Check sheet for the modelled part. Datum: model origin and axes. Units: mm. Face numbers are marked on the shaded views. A direction names the side the tool comes from. Round coordinates to 2 decimals unless told otherwise and drop trailing zeros. Write each loop counter-clockwise with the first axis right and the second up, starting at its lowest first coordinate (ties: lowest second). Pieces come first, ordered by that corner, then holes. Notation, with made-up numbers: (-31.5, -13.75) - (-15.5, -13.75) arc R13 cw to (-15.5, 6.25) - close; hole circle Ø2 at (-33, 21.5). An arc over 180 degrees is marked (long way). Use one line per item in the form item = value. Start each with the question number.
1) Section check D-D (y = 9.5). Record the boundary of the cut face in (x, z), then the cut area to 3 significant figures.
2) Scan lines: probe 1 along X at (y, z) = (21, 2.5); probe 2 along Y at (x, z) = (32, 6); probe 3 along X at (y, z) = (23.5, 4.75). Record each from-to range of solid material in increasing order.
3) Draft check along Y on the marked faces 1, 2 and 3. Enter one of: +Y half, -Y half, draft (parallel to the pull), parting line (faces both ways), or undercut.
4) Section check A-A (y = 3). Record the boundary of the cut face in (x, z).
5) Section check C-C (x = 28). Record the boundary of the cut face in (y, z), then the cut area to 3 significant figures.
6) Set-up check for the marked faces 4, 5, 6 and 7: record each of +Z, -Z, +X, -X, +Y, -Y from which the full face is reachable in a straight line by a thin tool's end or side.
7) Gauge pin test, flat ends, axial feed: P1, Ø1.5, axis at y = 33, z = 3, coming from the -X side; P2, Ø2.5, axis at y = 31.49, z = 5, coming from the +X side; P3, Ø2, axis at x = 26, z = 8, coming from the +Y side. Record the tip position at first contact, or that the pin passes through.
8) Section check B-B (x = 24). Record the boundary of the cut face in (y, z).
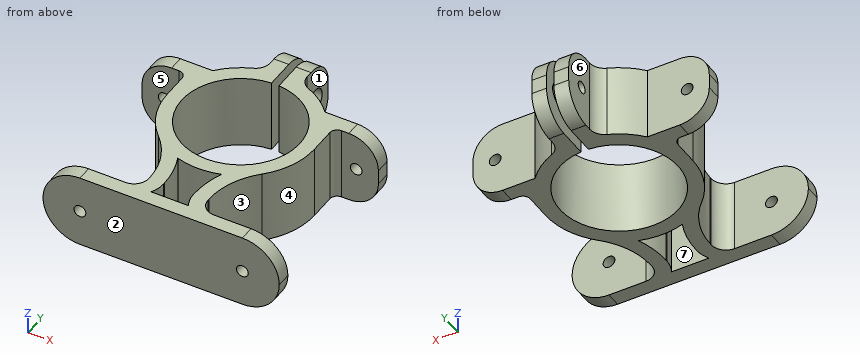
from build123d import *

# Parameters (mm, degrees)
BOSS_EXTRUDE1_DEPTH = 10
SKETCH3_R           = 0.8
CUT_EXTRUDE1_DEPTH  = 2
SKETCH4_R           = 0.8
CUT_EXTRUDE2_DEPTH  = 2
SKETCH5_R           = 0.8
CUT_EXTRUDE3_DEPTH  = 2
SKETCH6_R           = 0.8
CUT_EXTRUDE4_DEPTH  = 3
SKETCH7_R           = 1.6
CUT_EXTRUDE5_DEPTH  = 3
CUT_EXTRUDE6_DEPTH  = 10


with BuildPart() as part:
    # Sketch1 → Boss-Extrude1 (new body)
    with BuildSketch(Plane.XY):
        with BuildLine():
            Line((16.803004448, 0), (48.803096805, 0))
            Line((48.803096805, 0), (48.803096805, 2))
            Line((48.803096805, 2), (38.803096805, 2))
            ThreePointArc((38.803096805, 2), (37.388883243, 2.585786438), (36.803096805, 4))
            Line((36.803096805, 4), (36.803096805, 4.217123744))
            ThreePointArc((36.803096805, 4.217123744), (37.58355047, 8.090102619), (39.803089878, 11.358545383))
            ThreePointArc((39.803089878, 11.358545383), (42.022639537, 14.62700324), (42.803096805, 18.5))
            Line((42.803096805, 18.5), (42.803096805, 22))
            ThreePointArc((42.803096805, 22), (43.095990024, 22.707106781), (43.803096805, 23))
            Line((43.803096805, 23), (48.803096805, 23))
            Line((48.803096805, 23), (48.803096805, 25))
            Line((48.803096805, 25), (44.105786895, 25))
            Line((44.105786895, 25), (40.40245347, 25))
            ThreePointArc((40.40245347, 25), (38.644426823, 26.616603213), (36.553207437, 27.770234489))
            ThreePointArc((36.553207437, 27.770234489), (35.644914528, 28.506251313), (35.303235335, 29.624272825))
            Line((35.303235335, 29.624272825), (35.303235335, 34.487492178))
            Line((35.303235335, 34.487492178), (33.303050626, 34.487492178))
            Line((33.303050626, 34.487492178), (33.303050626, 26.484348185))
            ThreePointArc((33.303050626, 26.484348185), (32.803050626, 10.500011503), (32.303050626, 26.484348185))
            Line((32.303050626, 26.484348185), (32.303050626, 34.487492178))
            Line((32.303050626, 34.487492178), (30.303050626, 34.487492178))
            Line((30.303050626, 34.487492178), (30.303050626, 29.624347545))
            ThreePointArc((30.303050626, 29.624347545), (29.961362151, 28.506312265), (29.05304774, 27.770296755))
            ThreePointArc((29.05304774, 27.770296755), (26.961741815, 26.616651708), (25.203647783, 25))
            Line((25.203647783, 25), (21.500314358, 25))
            Line((21.500314358, 25), (16.803004448, 25))
            Line((16.803004448, 25), (16.803004448, 23))
            Line((16.803004448, 23), (21.803004448, 23))
            ThreePointArc((21.803004448, 23), (22.510111229, 22.707106781), (22.803004448, 22))
            Line((22.803004448, 22), (22.803004448, 18.5))
            ThreePointArc((22.803004448, 18.5), (23.583461716, 14.62700324), (25.803011375, 11.358545383))
            ThreePointArc((25.803011375, 11.358545383), (28.022550783, 8.090102619), (28.803004448, 4.217123744))
            Line((28.803004448, 4.217123744), (28.803004448, 4))
            ThreePointArc((28.803004448, 4), (28.21721801, 2.585786438), (26.803004448, 2))
            Line((26.803004448, 2), (16.803004448, 2))
            Line((16.803004448, 2), (16.803004448, 0))
        make_face()
        with BuildLine():
            Line((34.803096805, 4), (34.803096805, 4.217123744))
            ThreePointArc((34.803096805, 4.217123744), (35.049071096, 6.634328662), (35.776910074, 8.952438536))
            ThreePointArc((35.776910074, 8.952438536), (32.803050626, 8.500011503), (29.829191179, 8.952438536))
            ThreePointArc((29.829191179, 8.952438536), (30.557030157, 6.634328662), (30.803004448, 4.217123744))
            Line((30.803004448, 4.217123744), (30.803004448, 4))
            ThreePointArc((30.803004448, 4), (30.666707753, 2.96472382), (30.267106063, 2))
            Line((30.267106063, 2), (35.33899519, 2))
            ThreePointArc((35.33899519, 2), (34.9393935, 2.96472382), (34.803096805, 4))
        make_face(mode=Mode.SUBTRACT)
    extrude(amount=BOSS_EXTRUDE1_DEPTH)

    # Sketch3 → Cut-Extrude1 (cut)
    with BuildSketch(Plane(origin=(0, 2, 0), x_dir=(1, 0, 0), z_dir=(0, 1, 0))):
        with BuildLine():
            ThreePointArc((48.803096805, -5), (47.338630711, -8.535533906), (43.803096805, -10))
            Line((43.803096805, -10), (48.803096805, -10))
            Line((48.803096805, -10), (48.803096805, -5))
        make_face()
        with BuildLine():
            ThreePointArc((43.803096805, 0), (47.338630711, -1.464466094), (48.803096805, -5))
            Line((48.803096805, -5), (48.803096805, 0))
            Line((48.803096805, 0), (43.803096805, 0))
        make_face()
        with Locations(Location((43.803096805, -5, 0), (0, 0, 180))):
            Circle(SKETCH3_R)
    extrude(amount=-CUT_EXTRUDE1_DEPTH, mode=Mode.SUBTRACT)

    # Sketch4 → Cut-Extrude2 (cut)
    with BuildSketch(Plane(origin=(0, 2, 0), x_dir=(1, 0, 0), z_dir=(0, 1, 0))):
        with BuildLine():
            Line((16.803004448, -10), (21.803004448, -10))
            ThreePointArc((21.803004448, -10), (18.267470542, -8.535533906), (16.803004448, -5))
            Line((16.803004448, -5), (16.803004448, -10))
        make_face()
        with BuildLine():
            Line((16.803004448, 0), (16.803004448, -5))
            ThreePointArc((16.803004448, -5), (18.267470542, -1.464466094), (21.803004448, 0))
            Line((21.803004448, 0), (16.803004448, 0))
        make_face()
        with Locations(Location((21.803004448, -5, 0), (0, 0, 270))):
            Circle(SKETCH4_R)
    extrude(amount=-CUT_EXTRUDE2_DEPTH, mode=Mode.SUBTRACT)

    # Sketch5 → Cut-Extrude3 (cut)
    with BuildSketch(Plane(origin=(0, 25, 0), x_dir=(1, 0, 0), z_dir=(0, 1, 0))):
        with Locations(Location((19.803004448, -5, 0), (0, 0, 270))):
            Circle(SKETCH5_R)
        with Locations(Location((45.803096805, -5, 0), (0, 0, 270))):
            Circle(SKETCH5_R)
        with BuildLine():
            Line((20.803004448, -10), (16.803004448, -10))
            Line((16.803004448, -10), (16.803004448, -6))
            ThreePointArc((16.803004448, -6), (17.974577323, -8.828427125), (20.803004448, -10))
        make_face()
        with BuildLine():
            Line((16.803004448, -4), (16.803004448, 0))
            Line((16.803004448, 0), (20.803004448, 0))
            ThreePointArc((20.803004448, 0), (17.974577323, -1.171572875), (16.803004448, -4))
        make_face()
        with BuildLine():
            Line((44.803096805, 0), (48.803096805, 0))
            Line((48.803096805, 0), (48.803096805, -4))
            ThreePointArc((48.803096805, -4), (47.63152393, -1.171572875), (44.803096805, 0))
        make_face()
        with BuildLine():
            Line((48.803096805, -6), (48.803096805, -10))
            Line((48.803096805, -10), (44.803096805, -10))
            ThreePointArc((44.803096805, -10), (47.63152393, -8.828427125), (48.803096805, -6))
        make_face()
    extrude(amount=-CUT_EXTRUDE3_DEPTH, mode=Mode.SUBTRACT)

    # Sketch6 → Cut-Extrude4 (cut)
    with BuildSketch(Plane.ZY.offset(-30.303050626)):
        with Locations((5, 31.487492178)):
            Circle(SKETCH6_R)
    extrude(amount=-CUT_EXTRUDE4_DEPTH, mode=Mode.SUBTRACT)

    # Sketch7 → Cut-Extrude5 (cut)
    with BuildSketch(Plane(origin=(35.303235335, 0, 0), x_dir=(0, 0, -1), z_dir=(1, 0, 0))):
        with Locations((-5, 31.487492178)):
            Circle(SKETCH7_R)
    extrude(amount=-CUT_EXTRUDE5_DEPTH, mode=Mode.SUBTRACT)

    # Sketch8 → Cut-Extrude6 (cut)
    with BuildSketch(Plane.ZY.offset(-30.303050626)):
        with BuildLine():
            Line((0, 30.487492178), (0, 34.487492178))
            Line((0, 34.487492178), (4, 34.487492178))
            ThreePointArc((4, 34.487492178), (1.171572875, 33.315919302), (0, 30.487492178))
        make_face()
        with BuildLine():
            Line((6, 34.487492178), (10, 34.487492178))
            Line((10, 34.487492178), (10, 30.487492178))
            ThreePointArc((10, 30.487492178), (8.828427125, 33.315919302), (6, 34.487492178))
        make_face()
    extrude(amount=-CUT_EXTRUDE6_DEPTH, mode=Mode.SUBTRACT)


solid = part.part
Results are:
q1.outline = (27.29, 0) - (38.31, 0) - (38.31, 10) - (27.29, 10) - close
q1.area = 110 mm²
q2.probe_1 = 22.8 to 25.2, 40.4 to 42.8
q2.probe_2 = 0 to 2, 8.53 to 10.54, 26.46 to 34.49
q2.probe_3 = 16.8 to 19.04, 20.56 to 26.56, 39.05 to 45.04, 46.56 to 48.8
q3.face_1 = draft
q3.face_2 = -Y half
q3.face_3 = undercut
q4.outline = (28.54, 0) - (30.68, 0) - (30.68, 10) - (28.54, 10) - close; (34.93, 0) - (37.07, 0) - (37.07, 10) - (34.93, 10) - close
q5.outline = (0, 0) - (2.4, 0) - (2.4, 10) - (0, 10) - close; (8.14, 0) - (12.1, 0) - (12.1, 10) - (8.14, 10) - close; (24.9, 0) - (27.27, 0) - (27.27, 10) - (24.9, 10) - close
q5.area = 87.3 mm²
q6.face_4 = +Z, -Z, +X
q6.face_5 = +Z, -Z, -X
q6.face_6 = +Z, -Z, -X, +Y
q6.face_7 = +Z, -Z
q7.P1 = 30.3
q7.P2 = 32.3
q7.P3 = 26.64
q8.outline = (0, 0) - (2, 0) - (2, 10) - (0, 10) - close; (13.76, 0) - (25, 0) - (25, 10) - (13.76, 10) - close
